```python
from build123d import *

# Parameters (mm, degrees)
SKETCH1_W           = 50.292
SKETCH1_H           = 57.15
BOSS_EXTRUDE1_DEPTH = 3.175
SKETCH3_R           = 2.032
SKETCH3_R_2         = 1.984375
CUT_EXTRUDE1_DEPTH  = 4.175
CUT_EXTRUDE2_DEPTH  = 4.175
FILLET1_R           = 1.5875
BOSS_EXTRUDE2_DEPTH = 9.525


with BuildPart() as part:
    # Sketch1 → Boss-Extrude1 (new body)
    with BuildSketch(Plane.XY):
        with Locations((25.146, -28.575)):
            Rectangle(SKETCH1_W, SKETCH1_H)
    extrude(amount=BOSS_EXTRUDE1_DEPTH)

    # Sketch3 → Cut-Extrude1 (cut, through all)
    with BuildSketch(Plane.XY.offset(3.175)):
        with Locations((25.146, -5.08)):
            Circle(SKETCH3_R)
        with Locations((42.6085, -5.08)):
            Circle(SKETCH3_R_2)
        with Locations((7.6835, -5.08)):
            Circle(SKETCH3_R_2)
        Polygon((0, -57.15), (9.271, -57.15), (0, -50.8), align=None)
        Polygon((50.292, -50.8), (41.021, -57.15), (50.292, -57.15), align=None)
    extrude(amount=-CUT_EXTRUDE1_DEPTH, mode=Mode.SUBTRACT)

    # Sketch4 → Cut-Extrude2 (cut, through all)
    with BuildSketch(Plane.XY.offset(3.175)):
        with BuildLine():
            Line((21.17725, -5.145617642), (21.17725, -3.96875))
            ThreePointArc((21.17725, -3.96875), (22.339669962, -1.162419962), (25.146, 0))
            Line((25.146, 0), (7.62, 0))
            ThreePointArc((7.62, 0), (9.334782633, -0.389574524), (10.71291739, -1.481816429))
            Line((10.71291739, -1.481816429), (15.24, -7.112))
            ThreePointArc((15.24, -7.112), (16.21713524, -7.8392426), (17.36190992, -8.2553748))
            ThreePointArc((17.36190992, -8.2553748), (20.008184352, -7.606684967), (21.17725, -5.145617642))
        make_face()
        with BuildLine():
            Line((42.672, 0), (25.146, 0))
            ThreePointArc((25.146, 0), (27.952330038, -1.162419962), (29.11475, -3.96875))
            Line((29.11475, -3.96875), (29.11475, -5.145617642))
            ThreePointArc((29.11475, -5.145617642), (30.283815648, -7.606684967), (32.93009008, -8.2553748))
            ThreePointArc((32.93009008, -8.2553748), (34.07486476, -7.8392426), (35.052, -7.112))
            Line((35.052, -7.112), (39.57908261, -1.481816429))
            ThreePointArc((39.57908261, -1.481816429), (40.957217367, -0.389574524), (42.672, 0))
        make_face()
        with BuildLine():
            Line((50.292, 0), (42.672, 0))
            ThreePointArc((42.672, 0), (44.386782633, -0.389574524), (45.76491739, -1.481816429))
            Line((45.76491739, -1.481816429), (50.292, -7.112))
            Line((50.292, -7.112), (50.292, 0))
        make_face()
        with BuildLine():
            ThreePointArc((4.52708261, -1.481816429), (5.905217367, -0.389574524), (7.62, 0))
            Line((7.62, 0), (0, 0))
            Line((0, 0), (0, -7.112))
            Line((0, -7.112), (4.52708261, -1.481816429))
        make_face()
    extrude(amount=-CUT_EXTRUDE2_DEPTH, mode=Mode.SUBTRACT)

    # Fillet1
    fillet1_edges = [part.edges().sort_by_distance(p)[0] for p in [
        (0, -7.112, 1.5875),
        (0, -50.8, 1.5875),
        (9.271, -57.15, 1.5875),
        (41.021, -57.15, 1.5875),
        (50.292, -50.8, 1.5875),
        (50.292, -7.112, 1.5875),
    ]]
    fillet(fillet1_edges, radius=FILLET1_R)

    # Sketch6 → Boss-Extrude2 (add)
    with BuildSketch(Plane.XY.offset(3.175)):
        with BuildLine():
            Line((1.5875, -17.239611386), (1.5875, -49.126312385))
            ThreePointArc((1.5875, -49.126312385), (1.770672966, -49.86659735), (2.277921203, -50.436047428))
            Line((2.277921203, -50.436047428), (9.284630112, -55.235163118))
            ThreePointArc((9.284630112, -55.235163118), (9.786487736, -55.462944408), (10.33597995, -55.505414371))
            ThreePointArc((10.33597995, -55.505414371), (25.146, -54.784098787), (39.95602005, -55.505414371))
            ThreePointArc((39.95602005, -55.505414371), (40.505512264, -55.462944408), (41.007369888, -55.235163118))
            Line((41.007369888, -55.235163118), (48.014078797, -50.436047428))
            ThreePointArc((48.014078797, -50.436047428), (48.521327034, -49.86659735), (48.7045, -49.126312385))
            Line((48.7045, -49.126312385), (48.7045, -17.239611386))
            ThreePointArc((48.7045, -17.239611386), (48.318520542, -16.202063972), (47.348273684, -15.669048197))
            ThreePointArc((47.348273684, -15.669048197), (25.146, -14.043114413), (2.943726316, -15.669048197))
            ThreePointArc((2.943726316, -15.669048197), (1.973479458, -16.202063972), (1.5875, -17.239611386))
        make_face()
    extrude(amount=BOSS_EXTRUDE2_DEPTH)


solid = part.part
```
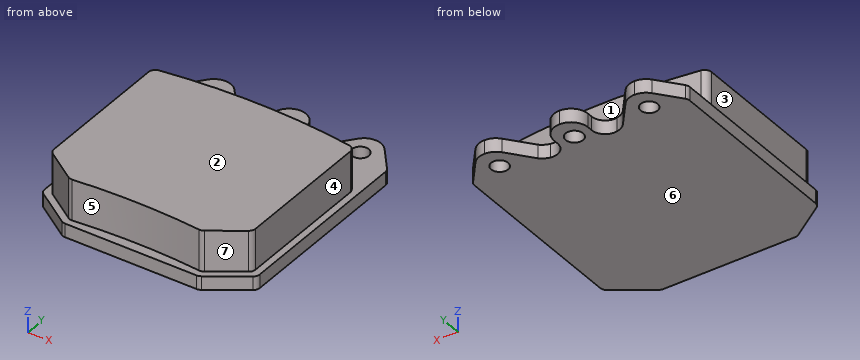
Input: part model. Units: mm. Frame: model coordinates. Face numbers are marked on the shaded views. A direction names the side the tool comes from. Give positions to 0.01 mm unless a question says otherwise; leave off trailing zeros. Write each loop counter-clockwise with the first axis right and the second up, starting at its lowest first coordinate (ties: lowest second). Pieces come first, ordered by that corner, then holes. Notation, with made-up numbers: (-32.5, -14.5) - (11.5, -14.5) arc R7 cw to (11.5, -3.5) - close; hole circle Ø5 at (-10.5, 49). An arc over 180 degrees is marked (long way). Write item = value, one per line. Start each with the question number.
1. Access query for the marked faces 1, 2, 3 and 4. Directions: +Z, -Z, +X, -X, +Y, -Y. A direction counts if a zero-diameter tool reaches every point of the face in a straight line with its end or side. Return the directions, or none.
2. Section query B-B, the plane z = 8.25. Output: boundary loops of the cut face in (x, y) (1 decimal), then the cut area to 3 significant figures.
3. Mould query, pull axis X, two halves, no side actions, for the marked faces 5, 6 and 7. Classes: released by +X, released by -X, zero draft, split by the parting line, or undercut.
4. Section query A-A, the plane z = 2. Count the separate pieces of the cut face and the enclosed holes in it, then the cut area to 3 significant figures.
5. First-contact query: pin 1 Ø4.5 at (x, y) = (42.61, -5.08) entering from +Z (3 decimals); pin 2 Ø1.5 at (x, z) = (7, 3.5) entering from -Y; pin 3 Ø3 at (x, y) = (7.68, -5.08) entering from +Z; pin 4 Ø0.9 at (y, z) = (-5, 1.5) entering from -X. Flat tips, straight axial feed; report the tip coordinate or a pass-through.
6. Section query D-D, the plane x = 30. Output: boundary loops of the cut face in (y, z) (3 decimals), then the cut area to 3 significant figures.
7. Ray query, L1, parallel to X at y = -41.5, z = 4; L2, parallel to Y at x = 23.5, z = 10.5. Return the intervals inside material, ascending.
8. Section query C-C, the plane y = -45. Output: boundary loops of the cut face in (x, z) (1 decimal).
Check sheet entries:
q1.face_1 = +Z, +Y
q1.face_2 = +Z, +X, -X, +Y, -Y
q1.face_3 = +Z, -X, +Y, -Y
q1.face_4 = +Z, +X, +Y, -Y
q2.outline = (1.6, -49.1) arc R1.6 ccw to (2.3, -50.4) - (9.3, -55.2) arc R1.6 ccw to (10.3, -55.5) arc R152.4 cw to (40, -55.5) arc R1.6 ccw to (41, -55.2) - (48, -50.4) arc R1.6 ccw to (48.7, -49.1) - (48.7, -17.2) arc R1.6 ccw to (47.3, -15.7) arc R152.4 ccw to (2.9, -15.7) arc R1.6 ccw to (1.6, -17.2) - close
q2.area = 1,860 mm2
q3.face_5 = undercut
q3.face_6 = zero draft
q3.face_7 = released by +X
q4.separate_pieces = 1
q4.enclosed_holes = 3
q4.area = 2,590 mm2
q5.pin_1 = 3.175
q5.pin_2 = -56.06
q5.pin_3 = through
q5.pin_4 = 1.34
q6.outline = (-57.15, 0) - (-7.345, 0) - (-7.345, 3.175) - (-14.12, 3.175) - (-14.12, 12.7) - (-54.861, 12.7) - (-54.861, 3.175) - (-57.15, 3.175) - close
q6.area = 546 mm2
q7.L1 = 1.59 to 48.7
q7.L2 = -54.79 to -14.05
q8.outline = (0, 0) - (50.3, 0) - (50.3, 3.2) - (48.7, 3.2) - (48.7, 12.7) - (1.6, 12.7) - (1.6, 3.2) - (0, 3.2) - close
